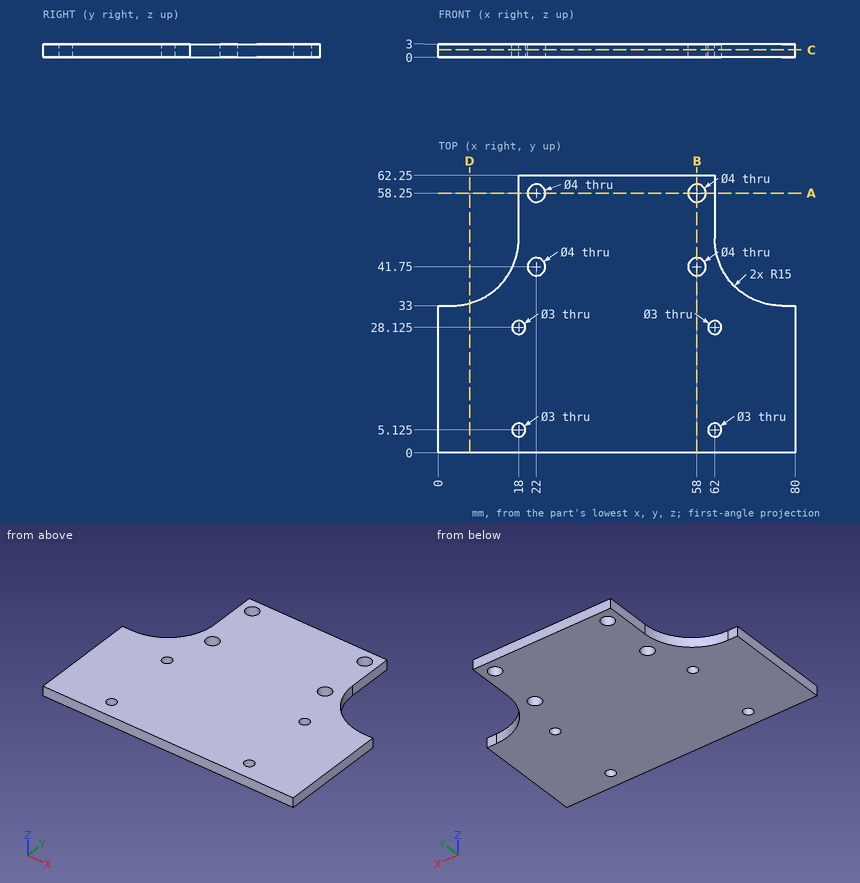
Can you work these out from the drawing? Everything is in mm from the part's minimum corner. Give positions to 0.01 mm unless a question says otherwise; leave off trailing zeros. Order: outer loops, then holes, each group sorted by start corner. A loop starts at its lowest first (then second) coordinate and runs counter-clockwise, first axis right, second up. Notation, with made-up numbers: M -4.75,0.5 L 17.25,0.5 A26 ccw 17.25,27.5 Z; hole C -11.5,74 d4. An arc over 180 degrees is marked long. Use a Markdown table: item, result. Add a question column.
1. I need wall thicknesses on probe 1 along X at (y, z) = (5, 2.15); probe 2 along X at (y, z) = (41, 1.2); probe 3 along X at (y, z) = (53, 0.35). Which ranges of each line are inside material? Lowest first, please. Write a range as from..to.
2. For pin 1 Ø1.5 at (x, z) = (78, 1.5) entering from +Y; pin 2 Ø1.8 at (x, y) = (62, 28.125) entering from -Z; pin 3 Ø1.5 at (x, z) = (14, 1) entering from +Y, each with a flat end and sliding along its axis, tell me the tip position at first contact or that it passes through.
3. Suppose I cut it at B-B (x = 58). List the corners of the cut face in (y, z) for me, and give its area (3 significant figures).
4. Suppose I cut it at A-A (y = 58.25). List the corners of the cut face in (x, z) for me.
5. Suppose I cut it at D-D (x = 7). List the corners of the cut face in (y, z) for me.
6. Suppose I cut it at C-C (z = 1.7). Give the number of separate pieces and of enclosed holes in the cut face, and give its area (3 significant figures).
Results list:
| question | item | result |
|---|---|---|
| 1 | probe 1 | x = 0..16.51, 19.49..60.51, 63.49..80 |
| 1 | probe 2 | x = 16.27..20.15, 23.85..56.15, 59.85..63.73 |
| 1 | probe 3 | x = 18..62 |
| 2 | pin 1 | stops at y = 33 |
| 2 | pin 2 | passes through |
| 2 | pin 3 | stops at y = 38.68 |
| 3 | outline | M 0,0 L 39.75,0 L 39.75,3 L 0,3 Z; M 43.75,0 L 56.25,0 L 56.25,3 L 43.75,3 Z; M 60.25,0 L 62.25,0 L 62.25,3 L 60.25,3 Z |
| 3 | area | 163 mm² |
| 4 | outline | M 18,0 L 20,0 L 20,3 L 18,3 Z; M 24,0 L 56,0 L 56,3 L 24,3 Z; M 60,0 L 62,0 L 62,3 L 60,3 Z |
| 5 | outline | M 0,0 L 33.54,0 L 33.54,3 L 0,3 Z |
| 6 | separate pieces | 1 |
| 6 | enclosed holes | 8 |
| 6 | area | 3,950 mm² |
